Check sheet for the modelled part. Datum: model origin and axes. Units: mm. A direction names the side the tool comes from. Coordinates: 2 decimals unless noted, no trailing zeros. Write each loop counter-clockwise with the first axis right and the second up, starting at its lowest first coordinate (ties: lowest second). Pieces come first, ordered by that corner, then holes. Notation, with made-up numbers: M 47.25,39 L 104.25,39 A29 ccw 104.25,76 Z; hole C 69,-20 d4. An arc over 180 degrees is marked long. Answer as CSV lines item,"result". Start each with the question number.
1) Material ranges on L1, parallel to Y at x = 14, z = 16.5; L2, parallel to X at y = 6, z = 4.5; L3, parallel to Z at x = 1.5, y = 7.75, recorded low to high. Write a range as [from, to].
2) Section check A-A (x = 6). Record the cut outline in (y, z), and give its area (3 significant figures).
3) Section check C-C (z = 27). Record the cut outline in (x, y).
4) Go/stop test with a flat-tipped pin: pin 1 Ø1 at (x, y) = (-2, -6) entering from -Z. Record where the tip stops, or that it passes through.
5) Draft check along X on faces 4 (the flat face through (-21.5, 0, 17)), 5 (the flat face through (0, 9, 19)), 6 (the flat face through (9, 0, 0)). Enter one of: +X half, -X half, draft (parallel to the pull), parting line (faces both ways), or undercut.
6) Section check D-D (y = -7.25). Record the cut outline in (x, z), and give its area (3 significant figures).
7) Access from +Z, -Z, +X, -X, +Y, -Y to the whole of each face (thin tool, end or side, straight path). Record for faces 1 (the flat face through (8, 0, 2)), 2 (the flat face through (-5, -6.215, 1)), 3 (the flat face through (21.5, 0, 17)).
8) Section check B-B (y = -4.75). Record the cut outline in (x, z).
from build123d import *

# Parameters (mm, degrees)
F0_W     = 43
F0_H     = 22
F1_DEPTH = 35
F2_W     = 39
F2_H     = 18
F3_DEPTH = 33
F4_W     = 24.357798
F4_H     = 12.429554
F5_DEPTH = 25


with BuildPart() as f1:
    # F0 (on Top) → F1 (new body)
    with BuildSketch(Plane.XY):
        Rectangle(F0_W, F0_H)
    extrude(amount=F1_DEPTH)

    # F2 (on face) → F3 (cut)
    with BuildSketch(Plane.XY.offset(35)):
        Rectangle(F2_W, F2_H)
    extrude(amount=-F3_DEPTH, mode=Mode.SUBTRACT)

    # F4 (on Top) → F5 (cut)
    with BuildSketch(Plane.XY):
        with Locations((-4.539045, 0)):
            Rectangle(F4_W, F4_H)
    extrude(amount=F5_DEPTH, mode=Mode.SUBTRACT)


solid = f1.part
Results found:
1,L1,"y = [-11, -9], [9, 11]"
1,L2,"x = [-21.5, -19.5], [19.5, 21.5]"
1,L3,"z = [0, 2]"
2,outline,"M -11,0 L -6.21,0 L -6.21,2 L -9,2 L -9,35 L -11,35 Z; M 6.21,0 L 11,0 L 11,35 L 9,35 L 9,2 L 6.21,2 Z"
2,area,"151 mm2"
3,outline,"M -21.5,-11 L 21.5,-11 L 21.5,11 L -21.5,11 Z; hole M -19.5,-9 L 19.5,-9 L 19.5,9 L -19.5,9 Z"
4,pin 1,"stops at z = 0"
5,face 4,"-X half"
5,face 5,"undercut"
5,face 6,"draft"
6,outline,"M -21.5,0 L 21.5,0 L 21.5,35 L 19.5,35 L 19.5,2 L -19.5,2 L -19.5,35 L -21.5,35 Z"
6,area,"218 mm2"
7,face 1,"+Z"
7,face 2,"+Z, -Z"
7,face 3,"+Z, -Z, +X, +Y, -Y"
8,outline,"M -21.5,0 L -16.72,0 L -16.72,2 L -19.5,2 L -19.5,35 L -21.5,35 Z; M 7.64,0 L 21.5,0 L 21.5,35 L 19.5,35 L 19.5,2 L 7.64,2 Z"
